Autodesk Fusion 360 part; units mm, degrees
sketch "Sketch1" plane through (0, 0, 0) normal (0, 1, 0) x (1, 0, 0)
  line L0 (0, 130) -> (0, -122.2085) construction
  line L1 (-100, 0) -> (125, 0) construction
  line L2 (40, 100) -> (-40, 100)
  line L3 (-40, 100) -> (-40, -100)
  line L4 (-40, -100) -> (40, -100)
  line L5 (40, -100) -> (40, 100)
  line L6 (40, 100) -> (-40, -100) construction
  line L7 (-40, 100) -> (40, -100) construction
  circle A0 centre (-28, -88) radius 3
  circle A1 centre (0, 0) radius 3
  circle A2 centre (-28, 88) radius 3
  circle A3 centre (28, 88) radius 3
  circle A4 centre (28, -88) radius 3
  dimension "d1" = 80
  dimension "d2" = 200
  dimension "d3" = 6
  dimension "d4" = 6
  dimension "d5" = 12
  dimension "d6" = 12
extrude "Extrude1" add sketch "Sketch1" along normal blind 12
fillet "Fillet1" radius 4 1 edges at (-2.797, 12, -1.0848)
fillet "Fillet2" radius 3.5 4 edges at (40, 6, -100) (-40, 6, -100) (-40, 6, 100) (40, 6, 100)
sketch "Sketch2" plane through (0, 0, 100) normal (0, 0, 1) x (1, 0, 0)
  line L0 (36.5, 0) -> (36.5, 12)
  line L1 (36.5, 12) -> (-36.5, 12)
  line L2 (-36.5, 12) -> (-36.5, 0)
  line L3 (-36.5, 0) -> (36.5, 0)
  line L4 (0, 12) -> (0, 0) construction
  line L5 (7, 12) -> (7, 0) construction
  line L6 (7, 12) -> (-7, 12) construction
  line L7 (25, 12) -> (31, 12) construction
  line L8 (25, 12) -> (25, 0) construction
  line L9 (25, 0) -> (7, 12) construction
  line L10 (7, 0) -> (25, 12) construction
  circle A0 centre (16, 6) radius 2.5
  dimension "d13" = 7
  dimension "d14" = 14
  dimension "d15" = 6
  dimension "d16" = 5
extrude "Extrude2" cut sketch "Sketch2" against normal blind 200 contours A0
equation "d6 = d5"
equation "d13 = d14 / 2"
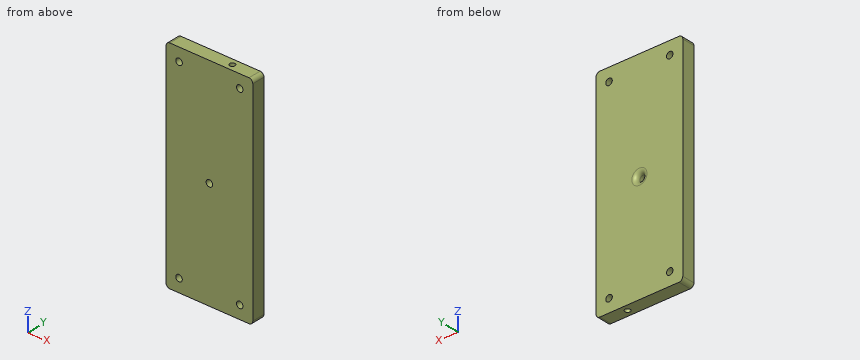
Geometry check sheet. Reference: the model listing, model coordinates, mm. Coordinates: 2 decimals unless noted, no trailing zeros. Order: outer loops, then holes, each group sorted by start corner. A loop starts at its lowest first (then second) coordinate and runs counter-clockwise, first axis right, second up. Notation, with made-up numbers: M -18.5,-27 L 26.5,-27 A23 cw 26.5,-13 Z; hole C 37.25,12 d5. An arc over 180 degrees is marked long. Answer as a JSON object with one key per item and string values.
Q1. Cross-section at C-C on x = 16. Record the cut outline in (y, z), and give its area (3 significant figures).
Results are:
{"outline": "M 0,-100 L 3.5,-100 L 3.5,100 L 0,100 Z; M 8.5,-100 L 12,-100 L 12,100 L 8.5,100 Z", "area": "1,400 mm²"}
Q2. Cross-section at B-B on x = 28. Record the cut outline in (y, z).
Results are:
{"outline": "M 0,-100 L 12,-100 L 12,-91 L 0,-91 Z; M 0,-85 L 12,-85 L 12,85 L 0,85 Z; M 0,91 L 12,91 L 12,100 L 0,100 Z"}
Q3. Cross-section at A-A on z = -88. Record the cut outline in (x, y), and give its area (3 significant figures).
Results are:
{"outline": "M -40,0 L -31,0 L -31,12 L -40,12 Z; M -25,0 L 25,0 L 25,12 L -25,12 Z; M 31,0 L 40,0 L 40,12 L 31,12 Z; hole C 16,6 d5", "area": "796 mm²"}
Q4. Depth check by flat-ended pin: pin 1 Ø5 at (x, z) = (-28, -88) entering from +Y; pin 2 Ø7 at (x, z) = (28, -88) entering from +Y. Enter the tip coordinate at first touch or a pass-through.
Results are:
{"pin 1": "passes through", "pin 2": "stops at y = 12"}
Q5. Scan lines: line 1 (Z direction, x = -28, y = 8.25); line 2 (X direction, y = 6.75, z = -1); line 3 (X direction, y = 6.5, z = 88). Record each from-to range of solid material in increasing order.
Results are:
{"line 1": "z = -100 to -91, -85 to 85, 91 to 100", "line 2": "x = -40 to -2.83, 2.83 to 13.62, 18.38 to 40", "line 3": "x = -40 to -31, -25 to 13.55, 18.45 to 25, 31 to 40"}
